The drawing under review shows one solid part. Ordinate dimensions are in mm from its lowest x, y, z. Coordinates: 2 decimals unless noted, no trailing zeros. Write each loop counter-clockwise with the first axis right and the second up, starting at its lowest first coordinate (ties: lowest second). Pieces come first, ordered by that corner, then holes.
1) Mouldability with a two-part tool opening along Y and no side actions: class the marked faces 1 and 2 as released by +Y, released by -Y, zero draft, split by the parting line, or undercut.
2) For line 1 (X direction, y = 0.5, z = 63.5) (1 decimal); line 2 (X direction, y = 11, z = 9.5) (1 decimal); line 3 (Y direction, x = 6, z = 13) (1 decimal), list the stretches that pass through material, from the lowest coordinate up.
3) For P1, Ø2, axis at y = 10.5, z = 52, coming from the +X side (1 decimal); P2, Ø3, axis at x = 6.5, z = 51.5, coming from the +Y side; P3, Ø4, axis at y = 7.5, z = 15.5, coming from the -X side; P4, Ø3, axis at x = 3.5, y = 2, coming from the -Z side, all flat-tipped, find the tip position at first contact; note any pin that passes through.
4) Add section A-A, the plane z = 59.5. State the section outline as (x, y) points (1 decimal).
5) Add section B-B, the plane x = 2.75. State the section outline as (y, z) points.
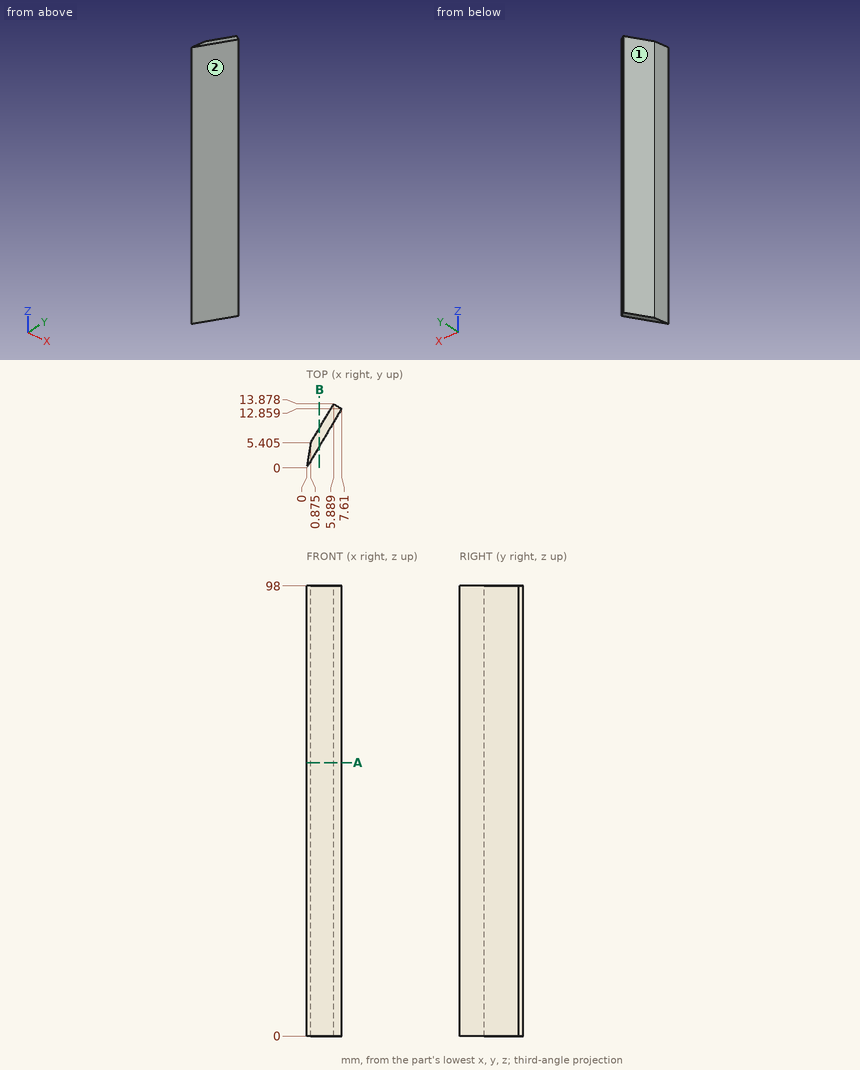
Geometry results:
1. face 1: released by +Y
1. face 2: released by -Y
2. line 1: x = 0.1 to 0.3
2. line 2: x = 4.2 to 6.5
2. line 3: y = 10.1 to 13.8
3. P1: stops at x = 6.8
3. P2: stops at y = 13.88
3. P3: stops at x = 0.93
3. P4: passes through
4. outline: (0, 0) - (7.6, 12.9) - (5.9, 13.9) - (0.9, 5.4) - close
5. outline: (4.65, 0) - (8.57, 0) - (8.57, 98) - (4.65, 98) - close
